from build123d import *

# Parameters (mm, degrees)
CHANFREIN1_SIZE         = 0.2
CONG_1_R                = 0.5
ESQUISSE3_W             = 0.767853135
ESQUISSE3_H             = 0.6
ENL_V_MAT_EXTRU_1_DEPTH = 5


with BuildPart() as part:
    # Esquisse1 → Base-Révolution (revolve)
    with BuildSketch(Plane.XY, mode=Mode.PRIVATE) as base_r_volution_sk:
        Polygon((-1.6, 0), (-1.6, 2.25), (0, 2.25), (0, 1.25), (10, 1.25), (10, 0), align=None)
    revolve(base_r_volution_sk.sketch.rotate(Axis((-28.982684825, 0, 0), (1, 0, 0)), 90), axis=Axis((-28.982684825, 0, 0), (1, 0, 0)))

    # Chanfrein1
    chanfrein1_edges = [part.edges().sort_by_distance(p)[0] for p in [
        (10, 0, -1.25),
    ]]
    chamfer(chanfrein1_edges, length=CHANFREIN1_SIZE)

    # Congé1
    cong_1_edges = [part.edges().sort_by_distance(p)[0] for p in [
        (-1.6, 0, -2.25),
    ]]
    fillet(cong_1_edges, radius=CONG_1_R)

    # Esquisse3 → Enlèv. mat.-Extru.1 (cut, symmetric)
    with BuildSketch(Plane.XY):
        with Locations((-1.383926568, 0)):
            Rectangle(ESQUISSE3_W, ESQUISSE3_H)
    extrude(amount=ENL_V_MAT_EXTRU_1_DEPTH, both=True, mode=Mode.SUBTRACT)


solid = part.part
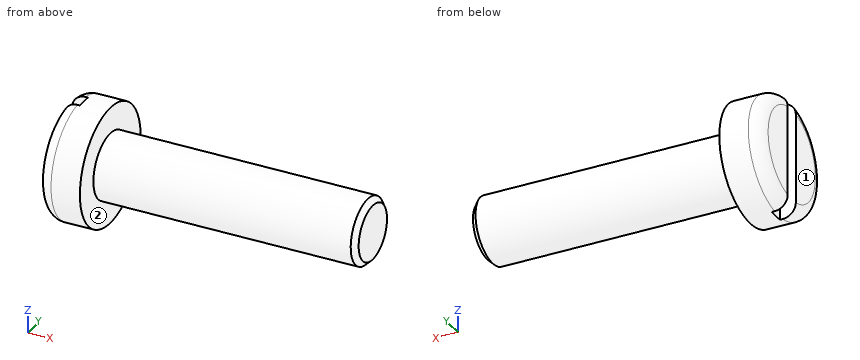
Could you check a few things on this model? Use its own coordinates, in mm. Face numbers are marked on the shaded views. A direction names the side the tool comes from. Give positions to 0.01 mm unless a question says otherwise; leave off trailing zeros. Loops run counter-clockwise (first coordinate to the right, second up) from the corner with the lowest first, then second, coordinate; pieces in that order, holes last. Notation, with made-up numbers: M -9,22.5 L -5,22.5 A15 cw -5,44.5 Z; hole C 70.25,-24.75 d11. An arc over 180 degrees is marked long. Answer as a JSON object with one key per item and string values.
Q1. Suppose I cut it at C-C, the plane x = -0.5. List the corners of the cut face in (y, z) for me, plus the area to 3 significant figures.
Values found:
{"outline": "C 0,0 d4.5", "area": "15.9 mm²"}
Q2. Suppose I cut it at B-B, the plane y = 0. List the corners of the cut face in (x, z) for me.
Values found:
{"outline": "M -1,-2.25 L 0,-2.25 L 0,-1.25 L 9.8,-1.25 L 10,-1.05 L 10,1.05 L 9.8,1.25 L 0,1.25 L 0,2.25 L -1,2.25 Z"}
Q3. Suppose I cut it at A-A, the plane z = 0. List the corners of the cut face in (x, y) for me, plus the area to 3 significant figures.
Values found:
{"outline": "M -1.6,-1.75 A0.5 ccw -1.1,-2.25 L 0,-2.25 L 0,-1.25 L 9.8,-1.25 L 10,-1.05 L 10,1.05 L 9.8,1.25 L 0,1.25 L 0,2.25 L -1.1,2.25 A0.5 ccw -1.6,1.75 L -1.6,0.3 L -1,0.3 L -1,-0.3 L -1.6,-0.3 Z", "area": "31.7 mm²"}
Q4. For the marked faces 1 and 2, which set-ups out of +Z, -Z, +X, -X, +Y, -Y let a thin tool reach every point of the face, with its end or its side?
Values found:
{"face 1": "+Z, -Z, -X, +Y, -Y", "face 2": "+X"}
Q5. For P1, Ø0.5, axis at y = 0, z = -1, coming from the -X side; P2, Ø2, axis at y = 1, z = -0.5, coming from the +X side; P3, Ø2, axis at x = 8, z = 1.5, coming from the +Y side; P4, Ø0.5, axis at x = -1.5, z = -1, coming from the -Y side, each with a flat end and sliding along its axis, tell me the tip position at first contact or that it passes through.
Values found:
{"P1": "stops at x = -1", "P2": "stops at x = 10", "P3": "stops at y = 1.15", "P4": "stops at y = -2.04"}
Q6. If I drill on probe 1 along X at (y, z) = (0.1, 0.1); probe 2 along X at (y, z) = (-1.3, 0.65); probe 3 along Y at (x, z) = (1.75, 0.15), over which ranges is the centre line in solid material (lowest first)? Write a range as [from, to].
Values found:
{"probe 1": "x = [-1, 10]", "probe 2": "x = [-1.6, 0]", "probe 3": "y = [-1.24, 1.24]"}
Q7. Suppose I cut it at D-D, the plane x = 5.25. List the corners of the cut face in (y, z) for me.
Values found:
{"outline": "C 0,0 d2.5"}
